Check sheet for the drawn part. Datum: minimum x, y, z corner. Units: mm. A direction names the side the tool comes from. Coordinates: 2 decimals unless noted, no trailing zeros. Order: outer loops, then holes, each group sorted by start corner. A loop starts at its lowest first (then second) coordinate and runs counter-clockwise, first axis right, second up.
1. Cross-section at B-B (y = 12). Enter the section's corners in (x, z), then the cut area to 3 significant figures.
2. Draft check along Z on the marked faces 5, 6 and 7. Enter one of: released by +Z, released by -Z, zero draft, split by the parting line, or undercut.
3. Gauge pin test, flat ends, axial feed: pin 1 Ø2.5 at (x, y) = (6, 10) entering from +Z; pin 2 Ø2 at (y, z) = (14.5, 29) entering from -X; pin 3 Ø2.5 at (x, z) = (5.5, 16.5) entering from +Y; pin 4 Ø3 at (x, y) = (6, 12) entering from -Z. Record the tip position at first contact, or that the pin passes through.
4. Cross-section at C-C (x = 6.5). Enter the section's corners in (y, z), then the cut area to 3 significant figures.
5. Set-up check for the marked faces 1, 2, 3 and 4: record each of +Z, -Z, +X, -X, +Y, -Y from which the full face is reachable in a straight line by a thin tool's end or side.
6. Cross-section at D-D (z = 23). Enter the section's corners in (x, y).
7. Cross-section at A-A (y = 6.5). Enter the section's corners in (x, z).
8. Thickness scan on line 1 (Y direction, x = 6, z = 28.75); line 2 (Z direction, x = 8, y = 13.25); line 3 (Y direction, x = 6, z = 1.8). Record the ranges inside material, lowest first.
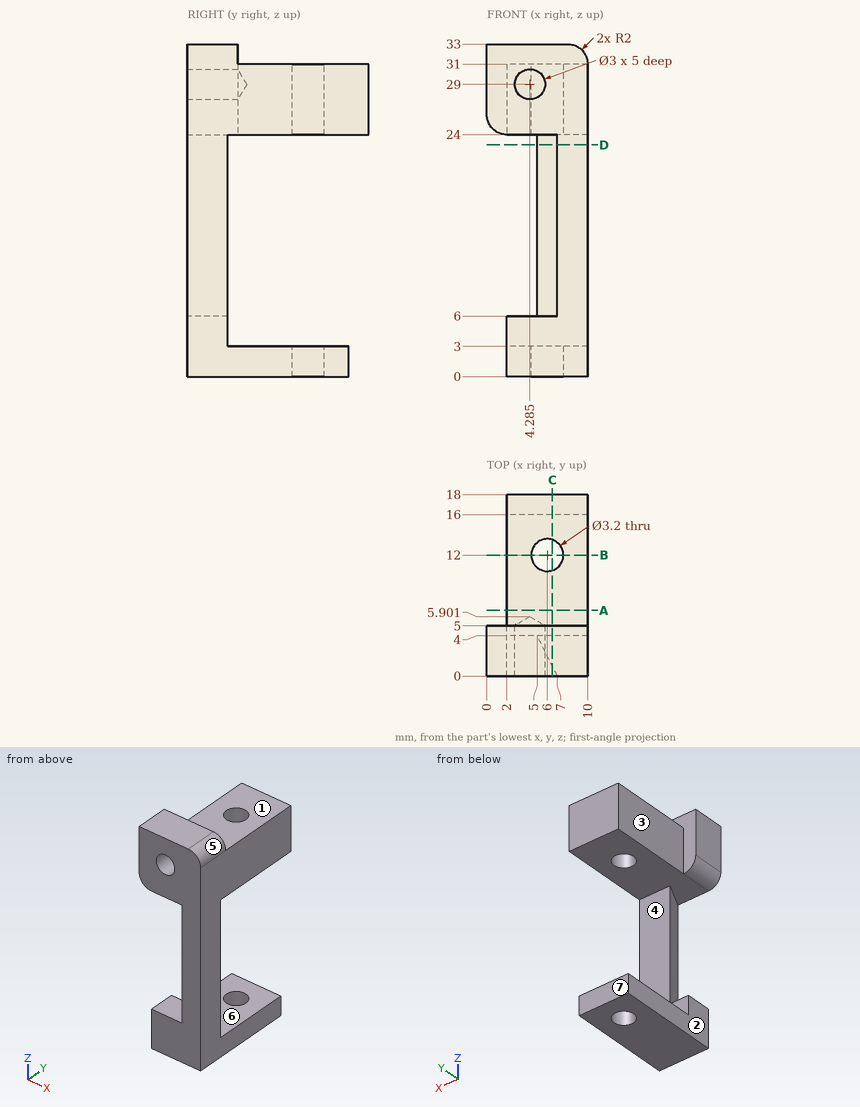
Data:
1. outline: (2, 0) - (4.4, 0) - (4.4, 3) - (2, 3) - close; (2, 24) - (4.4, 24) - (4.4, 31) - (2, 31) - close; (7.6, 0) - (10, 0) - (10, 3) - (7.6, 3) - close; (7.6, 24) - (10, 24) - (10, 31) - (7.6, 31) - close
1. area: 48.0 mm2
2. face 5: released by +Z
2. face 6: undercut
2. face 7: zero draft
3. pin 1: stops at z = 31
3. pin 2: stops at x = 2
3. pin 3: stops at y = 4
3. pin 4: passes through
4. outline: (0, 0) - (10.48, 0) - (10.48, 3) - (4, 3) - (4, 24) - (10.48, 24) - (10.48, 31) - (5, 31) - (5, 33) - (0, 33) - (0, 24) - (1, 24) - (1, 6) - (0, 6) - close; (13.52, 0) - (16, 0) - (16, 3) - (13.52, 3) - close; (13.52, 24) - (18, 24) - (18, 31) - (13.52, 31) - close
4. area: 220 mm2
5. face 1: +Z, +X, -X, +Y
5. face 2: -Z, -X, +Y, -Y
5. face 3: +Z, -Z, -X, +Y
5. face 4: +X, -X, +Y
6. outline: (5, 4) - (7, 0) - (10, 0) - (10, 4) - close
7. outline: (2, 0) - (10, 0) - (10, 3) - (2, 3) - close; (2, 24) - (10, 24) - (10, 31) - (2, 31) - close
8. line 1: y = 0 to 10.4, 13.6 to 18
8. line 2: z = 0 to 3, 24 to 31
8. line 3: y = 0 to 10.4, 13.6 to 16
